Check sheet for the modelled part. Datum: model origin and axes. Units: mm. A direction names the side the tool comes from. Give positions to 0.01 mm unless a question says otherwise; leave off trailing zeros. Loops run counter-clockwise (first coordinate to the right, second up) from the corner with the lowest first, then second, coordinate; pieces in that order, holes last. Notation, with made-up numbers: M 13,24 L 56,24 A30 ccw 56,50 Z; hole C 66.25,0.25 d7. An arc over 180 degrees is marked long. Use one line per item in the form item = value.
Autodesk Inventor part; units mm, degrees
ref_plane "YZ Plane" through (0, 0, 0) normal (1, 0, 0) x (0, 1, 0)
ref_plane "XZ Plane" through (0, 0, 0) normal (0, 1, 0) x (-1, 0, 0)
ref_plane "XY Plane" through (0, 0, 0) normal (0, 0, 1) x (1, 0, 0)
sketch "Sketch1" plane through (0, 0, 0) normal (0, 1, 0) x (-1, 0, 0)
  line L0 (26.4286, 13.8687) -> (-23.5714, 13.8687)
  line L1 (-23.5714, 13.8687) -> (-23.5714, -6.1313)
  line L2 (-23.5714, -6.1313) -> (-5.5714, -6.1313)
  line L3 (-5.5714, -6.1313) -> (-8.5714, -3.1313)
  line L4 (-8.5714, -3.1313) -> (11.4286, -3.1313)
  line L5 (11.4286, -3.1313) -> (8.4286, -6.1313)
  line L6 (8.4286, -6.1313) -> (26.4286, -6.1313)
  line L7 (26.4286, -6.1313) -> (26.4286, 13.8687)
  point P0 (0, 0)
  dimension "d0" = 50
  dimension "d15" = 20
  dimension "d16" = 3
  dimension "d17" = 45
  dimension "d22" = 20
extrude "Extrusion1" add sketch "Sketch1" along normal blind 20
sketch "Sketch2" plane through (23.5714, 0, 13.8687) normal (1, 0, 0) x (0, 0, -1)
  line L0 (0, 0) -> (0, 20)
  line L1 (0, 16.5) -> (8, 16.5)
  line L2 (8, 16.5) -> (8, 3.5)
  line L3 (8, 3.5) -> (0, 3.5)
  line L4 (0, 3.5) -> (0, 16.5)
  line L5 (0, 20) -> (20, 20)
  line L6 (5.2007, 20) -> (5.2007, 16.5) construction
  line L7 (5.2007, 3.5) -> (5.2007, 0) construction
  line L8 (0, 0) -> (20, 0)
  point P0 (13.8687, 0)
  dimension "d5" = 8
  dimension "d6" = 13
extrude "Extrusion2" cut sketch "Sketch2" against normal through all
sketch "Sketch3" plane through (0, 20, 0) normal (0, 1, 0) x (1, 0, 0)
  circle A0 centre (-20.9015, -9.3037) radius 2
  circle A1 centre (-7.6759, -9.3037) radius 2
  circle A2 centre (5.5497, -9.3037) radius 2
  circle A3 centre (18.7753, -9.3037) radius 2
  line L0 (-20.9015, -9.3037) -> (-7.6759, -9.3037) construction
  line L1 (-7.6759, -9.3037) -> (5.5497, -9.3037) construction
  line L2 (5.5497, -9.3037) -> (18.7753, -9.3037) construction
  point P0 (0, 0)
  dimension "d9" = 4
  dimension "d10" = 4
  dimension "d11" = 4
  dimension "d12" = 4
extrude "Extrusion3" cut sketch "Sketch3" against normal blind 5
fillet "Fillet1" radius 0.5 26 edges at (-26.4286, 18.25, 13.8687) (-26.4286, 20, 3.8687) (-26.4286, 10, -6.1313) (-26.4286, 0, 3.8687) (-26.4286, 1.75, 13.8687) (23.5714, 18.25, 13.8687) (-1.4286, 20, 13.8687) (23.5714, 1.75, 13.8687) (23.5714, 0, 3.8687) (23.5714, 10, -6.1313) (23.5714, 20, 3.8687) (-17.4286, 0, -6.1313) (-17.4286, 20, -6.1313) (-8.4286, 10, -6.1313) (-9.9286, 0, -4.6313) (-9.9286, 20, -4.6313) (-11.4286, 10, -3.1313) (-1.4286, 0, -3.1313) (-1.4286, 20, -3.1313) (8.5714, 10, -3.1313) (7.0714, 0, -4.6313) (7.0714, 20, -4.6313) (5.5714, 10, -6.1313) (14.5714, 0, -6.1313) (14.5714, 20, -6.1313) (-1.4286, 0, 13.8687)
sketch "Sketch4" plane through (0, 20, 0) normal (0, 1, 0) x (1, 0, 0)
  circle A0 centre (0, -2.9802) radius 2
  point P0 (0, 0)
  dimension "d19" = 4
extrude "Extrusion4" cut sketch "Sketch4" against normal through all
properties part number "Turning and Facing Holder"
1) Scan lines: line 1 (Y direction, x = 0.5, z = 7.25); line 2 (Z direction, x = 0, y = 6.25); line 3 (Z direction, x = -22, y = 10.25). Record each from-to range of solid material in increasing order.
Evaluation:
line_1 = 0 to 3.5, 16.5 to 20
line_2 = -3.13 to 0.98, 4.98 to 5.87
line_3 = -6.13 to 5.87
2) Section check A-A (x = 0). Record the cut outline in (y, z), then the cut area to 3 significant figures.
Evaluation:
outline = M 0,-2.63 A0.5 ccw 0.5,-3.13 L 19.5,-3.13 A0.5 ccw 20,-2.63 L 20,0.98 L 0,0.98 Z; M 0,4.98 L 20,4.98 L 20,13.37 A0.5 ccw 19.5,13.87 L 16.5,13.87 L 16.5,5.87 L 3.5,5.87 L 3.5,13.87 L 0.5,13.87 A0.5 ccw 0,13.37 Z
area = 156 mm^2
3) Release check for a two-part mould opening along X. For faces 5 (the face through (-1, 3.5, 10)), 6 (the face through (23.571, 10, 2)), 7 (the face through (1.908, 10.14, 2.379)) record: pulls with the +X half, pulls with the -X half, needs draft (parallel to the pull), parting line crosses it, or undercut.
Evaluation:
face_5 = needs draft
face_6 = pulls with the +X half
face_7 = undercut
4) Depth check by flat-ended pin: pin 1 Ø3.5 at (x, z) = (5.55, 9.3) entering from +Y; pin 2 Ø6 at (x, y) = (-8.5, 10) entering from +Z. Enter the tip coordinate at first touch or a pass-through.
Evaluation:
pin_1 = 3.5
pin_2 = 5.87
5) Set-up check for faces 1 (the face through (-2, 18, 13.869)), 2 (the face through (7.181, 0.15, -4.723)), 3 (the face through (17.19, 18.27, 10.52)), 4 (the face through (-9.94, 9.87, -4.62)): record each of +Z, -Z, +X, -X, +Y, -Y from which the full face is reachable in a straight line by a thin tool's end or side.
Evaluation:
face_1 = +Z, +X, -X, +Y, -Y
face_2 = -Y
face_3 = +Y
face_4 = +Y, -Y
6) Section check B-B (x = 9). Record the cut outline in (y, z), then the cut area to 3 significant figures.
Evaluation:
outline = M 0,-5.63 A0.5 ccw 0.5,-6.13 L 19.5,-6.13 A0.5 ccw 20,-5.63 L 20,13.37 A0.5 ccw 19.5,13.87 L 16.5,13.87 L 16.5,5.87 L 3.5,5.87 L 3.5,13.87 L 0.5,13.87 A0.5 ccw 0,13.37 Z
area = 296 mm^2
7) Section check C-C (y = 1). Record the cut outline in (x, z).
Evaluation:
outline = M -26.43,-5.63 A0.5 ccw -25.93,-6.13 L -9.64,-6.13 A0.5 ccw -9.28,-5.28 L -10.58,-3.98 A0.5 cw -10.22,-3.13 L 7.36,-3.13 A0.5 cw 7.72,-3.98 L 6.42,-5.28 A0.5 ccw 6.78,-6.13 L 23.07,-6.13 A0.5 ccw 23.57,-5.63 L 23.57,13.37 A0.5 ccw 23.07,13.87 L -25.93,13.87 A0.5 ccw -26.43,13.37 Z; hole C 0,2.98 d4
8) Section check D-D (z = 10.5). Record the cut outline in (x, y), then the cut area to 3 significant figures.
Evaluation:
outline = M -26.43,0.5 A0.5 ccw -25.93,0 L 23.07,0 A0.5 ccw 23.57,0.5 L 23.57,3.5 L -26.43,3.5 Z; M -26.43,16.5 L -22.5,16.5 L -22.5,20 L -25.93,20 A0.5 ccw -26.43,19.5 Z; M -19.3,16.5 L -9.28,16.5 L -9.28,20 L -19.3,20 Z; M -6.07,16.5 L 3.95,16.5 L 3.95,20 L -6.07,20 Z; M 7.15,16.5 L 17.17,16.5 L 17.17,20 L 7.15,20 Z; M 20.38,16.5 L 23.57,16.5 L 23.57,19.5 A0.5 ccw 23.07,20 L 20.38,20 Z
area = 305 mm^2
